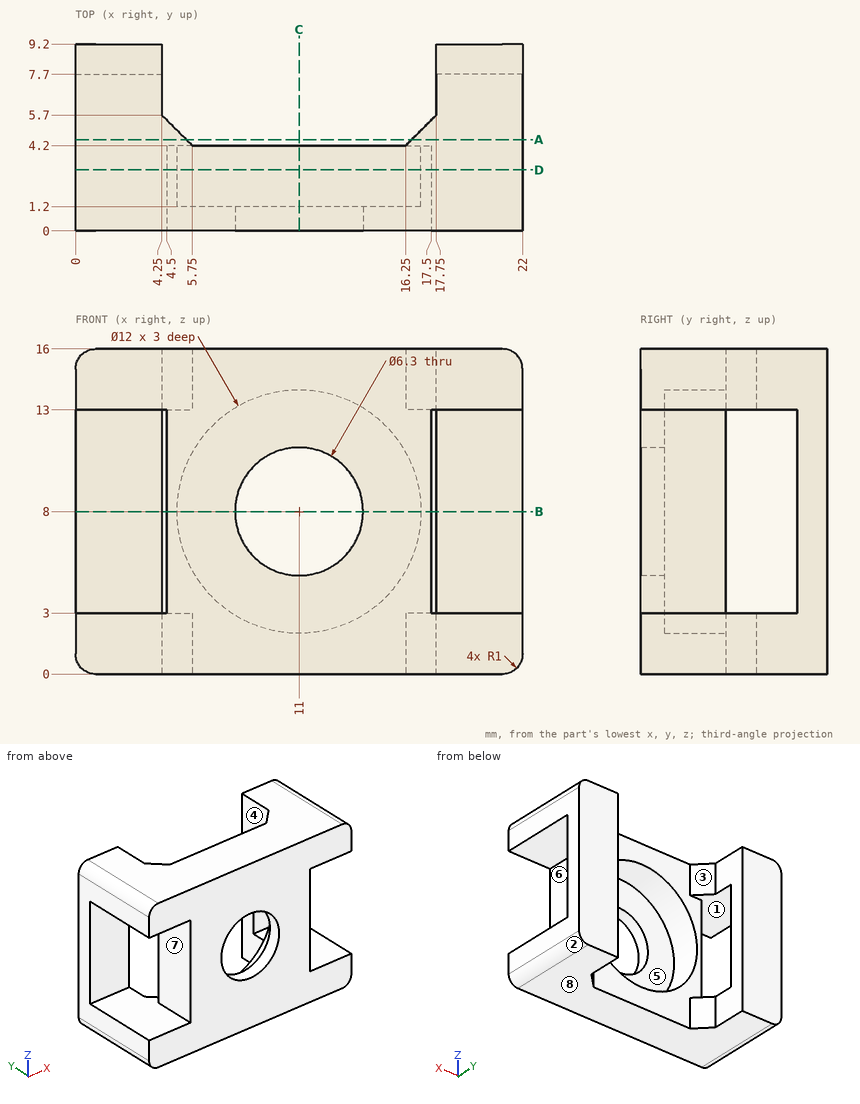
Geometry: see drawing. Coordinates: mm, zero at the bounding-box minimum. A direction names the side the tool comes from. Coordinates: 2 decimals unless noted, no trailing zeros. Write each loop counter-clockwise with the first axis right and the second up, starting at its lowest first coordinate (ties: lowest second). Pieces come first, ordered by that corner, then holes.
1) Mould query, pull axis Z, two halves, no side actions, for the marked faces 1, 2 and 3. Classes: pulls with the +Z half, pulls with the -Z half, needs draft (parallel to the pull), parting line crosses it, or undercut.
2) Section D-D on y = 3. Output: boundary loops of the cut face in (x, z).
3) Section C-C on x = 11. Output: boundary loops of the cut face in (y, z).
4) Section A-A on y = 4.5. Output: boundary loops of the cut face in (x, z).
5) Section B-B on z = 8. Output: boundary loops of the cut face in (x, y).
6) Set-up query: the marked faces 4, 5, 6, 7 and 8. Return all of +Z, -Z, +X, -X, +Y, -Y with unobstructed straight access to the full face (end or side cutting, diameter ignored); none if empty.
7) Pin query (flat end, axial travel): pin 1 Ø3.5 at (y, z) = (1.5, 7.5) entering from +X; pin 2 Ø3.5 at (x, z) = (1.5, 7.5) entering from -Y; pin 3 Ø8 at (x, z) = (9, 10.5) entering from +Y. Return the tip coordinate at first contact, or that it passes through.
8) Material intervals for line 1 along Z through (x, y) = (11, 0.35); line 2 along Z through (x, y) = (11, 2.8); line 3 along X through (y, z) = (8.5, 8.75), sorted ascending.
Check result:
1. face 1: undercut
1. face 2: pulls with the -Z half
1. face 3: needs draft
2. outline: (0, 1) arc R1 ccw to (1, 0) - (21, 0) arc R1 ccw to (22, 1) - (22, 3) - (17.5, 3) - (17.5, 13) - (22, 13) - (22, 15) arc R1 ccw to (21, 16) - (1, 16) arc R1 ccw to (0, 15) - (0, 13) - (4.5, 13) - (4.5, 3) - (0, 3) - close; hole circle Ø12 at (11, 8)
3. outline: (0, 0) - (4.2, 0) - (4.2, 2) - (1.2, 2) - (1.2, 4.85) - (0, 4.85) - close; (0, 11.15) - (1.2, 11.15) - (1.2, 14) - (4.2, 14) - (4.2, 16) - (0, 16) - close
4. outline: (0, 1) arc R1 ccw to (1, 0) - (5.45, 0) - (5.45, 3) - (0, 3) - close; (0, 13) - (5.45, 13) - (5.45, 16) - (1, 16) arc R1 ccw to (0, 15) - close; (16.55, 0) - (21, 0) arc R1 ccw to (22, 1) - (22, 3) - (16.55, 3) - close; (16.55, 13) - (22, 13) - (22, 15) arc R1 ccw to (21, 16) - (16.55, 16) - close
5. outline: (0, 7.7) - (4.25, 7.7) - (4.25, 9.2) - (0, 9.2) - close; (4.5, 0) - (7.85, 0) - (7.85, 1.2) - (5, 1.2) - (5, 4.2) - (4.5, 4.2) - close; (14.15, 0) - (17.5, 0) - (17.5, 4.2) - (17, 4.2) - (17, 1.2) - (14.15, 1.2) - close; (17.75, 7.7) - (22, 7.7) - (22, 9.2) - (17.75, 9.2) - close
6. face 4: +Z, -Z, +Y
6. face 5: +Y
6. face 6: +X, +Y, -Y
6. face 7: -X, +Y, -Y
6. face 8: -Z, +X, -X, +Y, -Y
7. pin 1: stops at x = 17.5
7. pin 2: stops at y = 7.7
7. pin 3: stops at y = 4.2
8. line 1: z = 0 to 4.85, 11.15 to 16
8. line 2: z = 0 to 2, 14 to 16
8. line 3: x = 0 to 4.25, 17.75 to 22
